from build123d import *

# Parameters (mm, degrees)
SKETCH1_W           = 85
SKETCH1_H           = 25
BOSS_EXTRUDE1_DEPTH = 6.3
SKETCH2_R           = 3.15
CUT_EXTRUDE1_DEPTH  = 45.745837795
SKETCH3_R           = 4.95
SKETCH3_W           = 45
SKETCH3_H           = 17.4
CUT_EXTRUDE3_DEPTH  = 1.5
SKETCH4_R           = 0.6
CUT_EXTRUDE4_DEPTH  = 45.745837795
SKETCH6_R           = 0.6
CUT_EXTRUDE5_DEPTH  = 45.745837795
SKETCH8_R           = 2.5
CUT_EXTRUDE6_DEPTH  = 3.2
CHAMFER1_SIZE       = 0.25


with BuildPart() as part:
    # Sketch1 → Boss-Extrude1 (new body)
    with BuildSketch(Plane.XY):
        Rectangle(SKETCH1_W, SKETCH1_H)
    extrude(amount=BOSS_EXTRUDE1_DEPTH)

    # Sketch2 → Cut-Extrude1 (cut, through all)
    with BuildSketch(Plane.XY.offset(6.3)):
        with Locations((32.55, 0)):
            Circle(SKETCH2_R)
        with Locations((-32.55, 0)):
            Circle(SKETCH2_R)
    extrude(amount=-CUT_EXTRUDE1_DEPTH, mode=Mode.SUBTRACT)

    # Sketch3 → Cut-Extrude3 (cut)
    with BuildSketch(Plane(origin=(0, 0, 0), x_dir=(-1, 0, 0), z_dir=(0, 0, -1))):
        Polygon((-45.439513652, -14.921110138), (-45.439513652, 15.191583433), (44.718251531, 15.191583433), (44.718251531, -15.912845555), align=None)
        with Locations((-32.55, 0)):
            Circle(SKETCH3_R, mode=Mode.SUBTRACT)
        with Locations((32.55, 0)):
            Circle(SKETCH3_R, mode=Mode.SUBTRACT)
        Rectangle(SKETCH3_W, SKETCH3_H, mode=Mode.SUBTRACT)
    extrude(amount=-CUT_EXTRUDE3_DEPTH, mode=Mode.SUBTRACT)

    # Sketch4 → Cut-Extrude4 (cut, through all)
    with BuildSketch(Plane.XY.offset(6.3)):
        with Locations((-1.1, -10.8)):
            Circle(SKETCH4_R)
        with Locations((1.1, -10.8)):
            Circle(SKETCH4_R)
        with Locations((-20.755, -10.8)):
            Circle(SKETCH4_R)
        with Locations((20.755, -10.8)):
            Circle(SKETCH4_R)
        with Locations((-1.1, -9.4)):
            Circle(SKETCH4_R)
        with Locations((1.1, -9.4)):
            Circle(SKETCH4_R)
        with Locations((20.755, -9.4)):
            Circle(SKETCH4_R)
        with Locations((-20.755, -9.4)):
            Circle(SKETCH4_R)
    extrude(amount=-CUT_EXTRUDE4_DEPTH, mode=Mode.SUBTRACT)

    # Sketch6 → Cut-Extrude5 (cut, through all)
    with BuildSketch(Plane.XY.offset(6.3)):
        with Locations((-20.825, 2.27)):
            Circle(SKETCH6_R)
        with Locations((21.575, 2.27)):
            Circle(SKETCH6_R)
    extrude(amount=-CUT_EXTRUDE5_DEPTH, mode=Mode.SUBTRACT)

    # Sketch8 → Cut-Extrude6 (cut)
    with BuildSketch(Plane.XY.offset(6.3)):
        with Locations((-20.825, 2.27)):
            Circle(SKETCH8_R)
        with Locations((21.575, 2.27)):
            Circle(SKETCH8_R)
        with BuildLine():
            Line((18.255, -12.5), (23.255, -12.5))
            Line((23.255, -12.5), (23.255, -9.4))
            ThreePointArc((23.255, -9.4), (20.755, -6.9), (18.255, -9.4))
            Line((18.255, -9.4), (18.255, -12.5))
        make_face()
        with BuildLine():
            Line((-1.1, -6.9), (1.1, -6.9))
            ThreePointArc((1.1, -6.9), (2.867766953, -7.632233047), (3.6, -9.4))
            Line((3.6, -9.4), (3.6, -12.5))
            Line((3.6, -12.5), (-3.6, -12.5))
            Line((-3.6, -12.5), (-3.6, -9.4))
            ThreePointArc((-3.6, -9.4), (-2.867766953, -7.632233047), (-1.1, -6.9))
        make_face()
        with BuildLine():
            Line((-23.255, -12.5), (-18.255, -12.5))
            Line((-18.255, -12.5), (-18.255, -9.4))
            ThreePointArc((-18.255, -9.4), (-20.755, -6.9), (-23.255, -9.4))
            Line((-23.255, -9.4), (-23.255, -12.5))
        make_face()
    extrude(amount=-CUT_EXTRUDE6_DEPTH, mode=Mode.SUBTRACT)

    # Chamfer1
    # the kernel refuses this chamfer: 0.25 mm, written as the material it takes off along each edge
    with BuildSketch(Plane(origin=(20.755, -9.4, 3.1), x_dir=(1, 0, 0), z_dir=(0, -1, 0))) as chamfer1_piece_1:
        Polygon((0.6, -CHAMFER1_SIZE), (0.6 + CHAMFER1_SIZE, 0), (0.6, 0), align=None)
    revolve(axis=Axis((20.755, -9.4, 3.1), (0, 0, 1)), mode=Mode.SUBTRACT)
    with BuildSketch(Plane(origin=(20.755, -10.8, 3.1), x_dir=(1, 0, 0), z_dir=(0, -1, 0))) as chamfer1_piece_2:
        Polygon((0.6, -CHAMFER1_SIZE), (0.6 + CHAMFER1_SIZE, 0), (0.6, 0), align=None)
    revolve(axis=Axis((20.755, -10.8, 3.1), (0, 0, 1)), mode=Mode.SUBTRACT)
    with BuildSketch(Plane(origin=(-20.825, 2.27, 3.1), x_dir=(1, 0, 0), z_dir=(0, -1, 0))) as chamfer1_piece_3:
        Polygon((0.6 + CHAMFER1_SIZE, 0), (0.6, -CHAMFER1_SIZE), (0.6, 0), align=None)
    revolve(axis=Axis((-20.825, 2.27, 3.1), (0, 0, 1)), mode=Mode.SUBTRACT)
    with BuildSketch(Plane(origin=(-20.755, -9.4, 3.1), x_dir=(1, 0, 0), z_dir=(0, -1, 0))) as chamfer1_piece_4:
        Polygon((0.6, -CHAMFER1_SIZE), (0.6 + CHAMFER1_SIZE, 0), (0.6, 0), align=None)
    revolve(axis=Axis((-20.755, -9.4, 3.1), (0, 0, 1)), mode=Mode.SUBTRACT)
    with BuildSketch(Plane(origin=(-20.755, -10.8, 3.1), x_dir=(1, 0, 0), z_dir=(0, -1, 0))) as chamfer1_piece_5:
        Polygon((0.6, -CHAMFER1_SIZE), (0.6 + CHAMFER1_SIZE, 0), (0.6, 0), align=None)
    revolve(axis=Axis((-20.755, -10.8, 3.1), (0, 0, 1)), mode=Mode.SUBTRACT)
    with BuildSketch(Plane(origin=(21.575, 2.27, 3.1), x_dir=(1, 0, 0), z_dir=(0, -1, 0))) as chamfer1_piece_6:
        Polygon((0.6 + CHAMFER1_SIZE, 0), (0.6, -CHAMFER1_SIZE), (0.6, 0), align=None)
    revolve(axis=Axis((21.575, 2.27, 3.1), (0, 0, 1)), mode=Mode.SUBTRACT)
    with BuildSketch(Plane(origin=(-1.1, -10.8, 3.1), x_dir=(1, 0, 0), z_dir=(0, -1, 0))) as chamfer1_piece_7:
        Polygon((0.6, -CHAMFER1_SIZE), (0.6 + CHAMFER1_SIZE, 0), (0.6, 0), align=None)
    revolve(axis=Axis((-1.1, -10.8, 3.1), (0, 0, 1)), mode=Mode.SUBTRACT)
    with BuildSketch(Plane(origin=(1.1, -9.4, 3.1), x_dir=(1, 0, 0), z_dir=(0, -1, 0))) as chamfer1_piece_8:
        Polygon((0.6, -CHAMFER1_SIZE), (0.6 + CHAMFER1_SIZE, 0), (0.6, 0), align=None)
    revolve(axis=Axis((1.1, -9.4, 3.1), (0, 0, 1)), mode=Mode.SUBTRACT)
    with BuildSketch(Plane(origin=(1.1, -10.8, 3.1), x_dir=(1, 0, 0), z_dir=(0, -1, 0))) as chamfer1_piece_9:
        Polygon((0.6, -CHAMFER1_SIZE), (0.6 + CHAMFER1_SIZE, 0), (0.6, 0), align=None)
    revolve(axis=Axis((1.1, -10.8, 3.1), (0, 0, 1)), mode=Mode.SUBTRACT)
    with BuildSketch(Plane(origin=(-1.1, -9.4, 3.1), x_dir=(1, 0, 0), z_dir=(0, -1, 0))) as chamfer1_piece_10:
        Polygon((0.6, -CHAMFER1_SIZE), (0.6 + CHAMFER1_SIZE, 0), (0.6, 0), align=None)
    revolve(axis=Axis((-1.1, -9.4, 3.1), (0, 0, 1)), mode=Mode.SUBTRACT)


solid = part.part
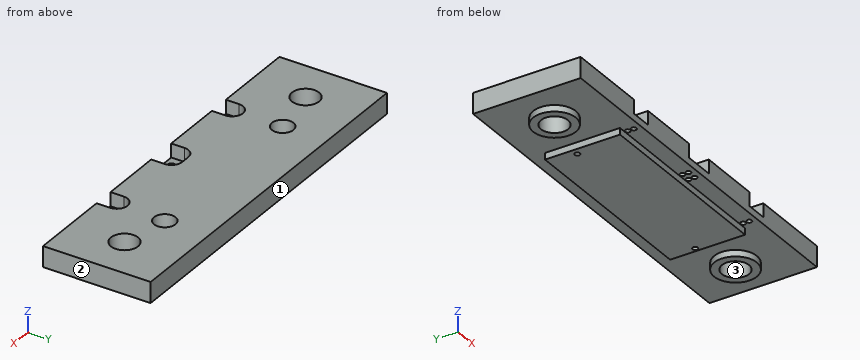
Verification items for the finished model (mm, model axes). Face numbers are marked on the shaded views. Coordinates: 2 decimals unless noted, no trailing zeros. Write each loop counter-clockwise with the first axis right and the second up, starting at its lowest first coordinate (ties: lowest second). Pieces come first, ordered by that corner, then holes. Notation, with made-up numbers: M 25,79 L 43,79 A23 cw 43,118 Z; hole C 32.5,76 d10. An arc over 180 degrees is marked long. Use a Markdown table: item, result.
Q1. Go/stop test with flat-tipped pins: P1, Ø1.8, axis at x = 0, z = 5, coming from the -Y side; P2, Ø0.7, axis at x = 1.1, y = -10.8, coming from the +Z side; P3, Ø1.6, axis at x = 2, z = 0.5, coming from the +Y side; P4, Ø1.7, axis at x = 0.5, y = -9, coming from the +Z side. Record where each tip stops, or that it passes through.
Reply:
| item | result |
|---|---|
| P1 | stops at y = -6.9 |
| P2 | passes through |
| P3 | stops at y = 8.7 |
| P4 | stops at z = 3.1 |
Q2. Sectioned sample at A-A, the plane x = -32.55. Record the boundary of the cut face in (y, z), plus the area to 3 significant figures.
Reply:
| item | result |
|---|---|
| outline | M -12.5,1.5 L -4.95,1.5 L -4.95,0 L -3.15,0 L -3.15,6.3 L -12.5,6.3 Z; M 3.15,0 L 4.95,0 L 4.95,1.5 L 12.5,1.5 L 12.5,6.3 L 3.15,6.3 Z |
| area | 95.2 mm² |
Q3. Thickness scan on line 1 (Y direction, x = -1.1, z = 1.9); line 2 (X direction, y = -10.75, z = 4.5) (3 decimals); line 3 (X direction, y = -9.5, z = 2). Record the ranges inside material, lowest first.
Reply:
| item | result |
|---|---|
| line 1 | y = -12.5 to -11.4, -10.2 to -10, -8.8 to 12.5 |
| line 2 | x = -42.5 to -23.255, -18.255 to -3.6, 3.6 to 18.255, 23.255 to 42.5 |
| line 3 | x = -42.5 to -21.35, -20.16 to -1.69, -0.51 to 0.51, 1.69 to 20.16, 21.35 to 42.5 |
Q4. Draft check along Y on the marked faces 1, 2 and 3. Enter one of: +Y half, -Y half, draft (parallel to the pull), parting line (faces both ways), or undercut.
Reply:
| item | result |
|---|---|
| face 1 | +Y half |
| face 2 | draft |
| face 3 | undercut |
Q5. Sectioned sample at B-B, the plane z = 4.5. Record the boundary of the cut face in (x, y) (3 decimals), plus the area to 3 significant figures.
Reply:
| item | result |
|---|---|
| outline | M -42.5,-12.5 L -23.255,-12.5 L -23.255,-9.4 A2.5 cw -18.255,-9.4 L -18.255,-12.5 L -3.6,-12.5 L -3.6,-9.4 A2.5 cw -1.1,-6.9 L 1.1,-6.9 A2.5 cw 3.6,-9.4 L 3.6,-12.5 L 18.255,-12.5 L 18.255,-9.4 A2.5 cw 23.255,-9.4 L 23.255,-12.5 L 42.5,-12.5 L 42.5,12.5 L -42.5,12.5 Z; hole C -32.55,0 d6.3; hole C -20.825,2.27 d5; hole C 21.575,2.27 d5; hole C 32.55,0 d6.3 |
| area | 1,940 mm² |
Q6. Sectioned sample at D-D, the plane y = -2. Record the boundary of the cut face in (x, z), plus the area to 3 significant figures.
Reply:
| item | result |
|---|---|
| outline | M -42.5,1.5 L -37.08,1.5 L -37.08,0 L -34.98,0 L -34.98,6.3 L -42.5,6.3 Z; M -30.12,0 L -28.02,0 L -28.02,1.5 L -22.5,1.5 L -22.5,0 L 22.5,0 L 22.5,1.5 L 28.02,1.5 L 28.02,0 L 30.12,0 L 30.12,6.3 L -30.12,6.3 Z; M 34.98,0 L 37.08,0 L 37.08,1.5 L 42.5,1.5 L 42.5,6.3 L 34.98,6.3 Z |
| area | 441 mm² |
Q7. Sectioned sample at C-C, the plane y = 6.75. Record the boundary of the cut face in (x, z).
Reply:
| item | result |
|---|---|
| outline | M -42.5,1.5 L -22.5,1.5 L -22.5,0 L 22.5,0 L 22.5,1.5 L 42.5,1.5 L 42.5,6.3 L -42.5,6.3 Z |
